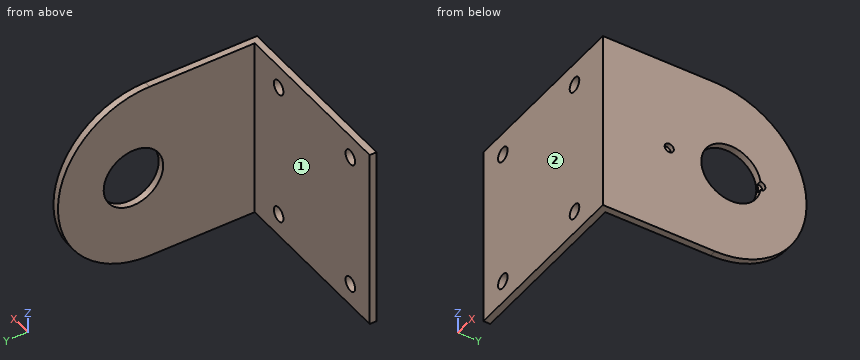
```python
from build123d import *

# Parameters (mm, degrees)
SKETCH_1_W          = 40
SKETCH_1_H          = 40
EXTRUDE_1_DEPTH     = 1.5
EXTRUDE_2_DEPTH     = 1.5
SKETCH_4_R          = 1.6
CUT_EXTRUDE_1_DEPTH = 45.5
SKETCH_6_R          = 6.5
CUT_EXTRUDE_2_DEPTH = 41
SKETCH_7_R          = 1
CUT_EXTRUDE_3_DEPTH = 1


with BuildPart() as part:
    # 草图1 → 凸台-拉伸1 (new body)
    with BuildSketch(Plane(origin=(0, 0, 0), x_dir=(1, 0, 0), z_dir=(0, 1, 0))):
        with Locations((-5, -7.5)):
            Rectangle(SKETCH_1_W, SKETCH_1_H)
    extrude(amount=EXTRUDE_1_DEPTH)

    # 草图3 → 凸台-拉伸2 (add)
    with BuildSketch(Plane(origin=(15, 0, 0), x_dir=(0, 0, -1), z_dir=(1, 0, 0))):
        with BuildLine():
            Line((-27.5, 1.5), (12.5, 1.5))
            Line((12.5, 1.5), (12.5, 24.5))
            ThreePointArc((12.5, 24.5), (-7.5, 44.5), (-27.5, 24.5))
            Line((-27.5, 24.5), (-27.5, 1.5))
        make_face()
    extrude(amount=-EXTRUDE_2_DEPTH)

    # 草图4 → 切除-拉伸1 (cut, through all)
    with BuildSketch(Plane.XZ):
        with Locations((-18.5, 22.5)):
            Circle(SKETCH_4_R)
        with Locations((-18.5, -7.5)):
            Circle(SKETCH_4_R)
        with Locations((5.5, 22.5)):
            Circle(SKETCH_4_R)
        with Locations((5.5, -7.5)):
            Circle(SKETCH_4_R)
    extrude(amount=-CUT_EXTRUDE_1_DEPTH, mode=Mode.SUBTRACT)

    # 草图6 → 切除-拉伸2 (cut, through all)
    with BuildSketch(Plane(origin=(15, 0, 0), x_dir=(0, 0, -1), z_dir=(1, 0, 0))):
        with Locations((-7.5, 28)):
            Circle(SKETCH_6_R)
    extrude(amount=-CUT_EXTRUDE_2_DEPTH, mode=Mode.SUBTRACT)

    # 草图7 → 切除-拉伸3 (cut)
    with BuildSketch(Plane(origin=(15, 0, 0), x_dir=(0, 0, -1), z_dir=(1, 0, 0))):
        with Locations((-7.5, 14.5)):
            Circle(SKETCH_7_R)
        with Locations((-7.5, 34.5)):
            Circle(SKETCH_7_R)
    extrude(amount=-CUT_EXTRUDE_3_DEPTH, mode=Mode.SUBTRACT)


solid = part.part
```
Design review of the part built by this model. Coordinates are the model's own, in mm. Face numbers are marked on the shaded views. A direction names the side the tool comes from. Give positions to 0.01 mm unless a question says otherwise; leave off trailing zeros. Order: outer loops, then holes, each group sorted by start corner. A loop starts at its lowest first (then second) coordinate and runs counter-clockwise, first axis right, second up. Notation, with made-up numbers: (35.5, 86) -> (85.5, 86) arc R26 ccw to (85.5, 121) -> close; hole circle Ø11 at (-20, 33.25). An arc over 180 degrees is marked (long way). Write each question's results on one line, items separated by ' | '. Start each with the question number.
Q1. Add section A-A on z = 7.5. Give the boundary of the cut face in (x, y).
Q2. For pin 1 (11.5 mm diameter, centred on x = -4, z = 5, fed in from +Y); pin 2 (10 mm diameter, centred on y = 17.5, z = 20.5, fed in from -X); pin 3 (1.2 mm diameter, centred on y = 14.5, z = 7.5, fed in from +X), all flat-tipped, find the tip position at first contact; note any pin that passes through.
Q3. Wall thickness on L1, parallel to Z at x = 5.5, y = 0.7; L2, parallel to Z at x = -18, y = 1; L3, parallel to X at y = 4.5, z = 3: over which ranges is each line inside the solid? List them lowest first. Write a range as from..to.
Q4. Machinability: for the marked faces 1 and 2, which of the approach directions +Z, -Z, +X, -X, +Y, -Y give a long, thin tool a straight path to every point of the face, cutting with its end or side? Answer none if there is none.
Q5. Add section D-D on z = -7.5. Give the boundary of the cut face in (x, y), and give its area (3 significant figures).
Q6. Add section B-B on x = -18.5. Give the boundary of the cut face in (y, z), and give its area (3 significant figures).
Q7. Add section C-C on y = 23. Give the boundary of the cut face in (x, z).
Found:
1) outline: (-25, 0) -> (15, 0) -> (15, 13.5) -> (14, 13.5) -> (14, 15.5) -> (15, 15.5) -> (15, 21.5) -> (13.5, 21.5) -> (13.5, 1.5) -> (-25, 1.5) -> close; (13.5, 34.5) -> (14, 34.5) -> (14, 35.5) -> (15, 35.5) -> (15, 44.5) -> (13.5, 44.5) -> close
2) pin 1: stops at y = 1.5 | pin 2: stops at x = 13.5 | pin 3: stops at x = 14
3) L1: z = -12.5..-9.1, -5.9..20.9, 24.1..27.5 | L2: z = -12.5..-9.02, -5.98..20.98, 24.02..27.5 | L3: x = 13.5..15
4) face 1: +Z, -Z, -X, +Y | face 2: +Z, -Z, +X, -X, -Y
5) outline: (-25, 0) -> (-20.1, 0) -> (-20.1, 1.5) -> (-25, 1.5) -> close; (-16.9, 0) -> (3.9, 0) -> (3.9, 1.5) -> (-16.9, 1.5) -> close; (7.1, 0) -> (15, 0) -> (15, 37.73) -> (13.5, 37.73) -> (13.5, 1.5) -> (7.1, 1.5) -> close | area: 105 mm2
6) outline: (0, -12.5) -> (1.5, -12.5) -> (1.5, -9.1) -> (0, -9.1) -> close; (0, -5.9) -> (1.5, -5.9) -> (1.5, 20.9) -> (0, 20.9) -> close; (0, 24.1) -> (1.5, 24.1) -> (1.5, 27.5) -> (0, 27.5) -> close | area: 50.4 mm2
7) outline: (13.5, -12.5) -> (15, -12.5) -> (15, 3.35) -> (13.5, 3.35) -> close; (13.5, 11.65) -> (15, 11.65) -> (15, 27.5) -> (13.5, 27.5) -> close
